from build123d import *

# Parameters (mm, degrees)
SKETCH1_W                     = 320
SKETCH1_H                     = 50
BOSS_EXTRUDE1_DEPTH           = 4
M5_CLEARANCE_HOLE1_AT_2_COUNT = 2
M5_CLEARANCE_HOLE1_AT_2_PITCH = 300
LPATTERN1_COUNT               = 2
LPATTERN1_PITCH               = 25
SKETCH5_W                     = 80
SKETCH5_H                     = 15
CUT_EXTRUDE1_DEPTH            = 324.907394173
CUT_EXTRUDE3_DEPTH            = 324.907394173
M2_5_CLEARANCE_HOLE1_D        = 2.9
M2_5_CLEARANCE_HOLE1_DEPTH    = 14
M2_5_CLEARANCE_HOLE1_TIP      = 0.871247898
DRAFT1_ANGLE                  = -20


with BuildPart() as part:
    # Sketch1 → Boss-Extrude1 (new body)
    with BuildSketch(Plane.XY):
        with Locations((160, 25)):
            Rectangle(SKETCH1_W, SKETCH1_H)
    extrude(amount=BOSS_EXTRUDE1_DEPTH)

    # Sketch4 → M5 Clearance Hole1 (revolve, cut)
    with BuildSketch(Plane(origin=(310, 37.5, 4), x_dir=(0, -1, 0), z_dir=(1, 0, 0))):
        Polygon((0, 0), (0, 15.652366702), (2.75, 14), (2.75, 0), align=None)
    m5_clearance_hole1 = revolve(axis=Axis((310, 37.5, 10.35), (0, 0, -1)), mode=Mode.SUBTRACT)

    # M5 Clearance Hole1 at 2: M5 Clearance Hole1 ×2
    with Locations(*[(-i * M5_CLEARANCE_HOLE1_AT_2_PITCH, 0, 0) for i in range(1, M5_CLEARANCE_HOLE1_AT_2_COUNT)]):
        add(m5_clearance_hole1, mode=Mode.SUBTRACT)

    # LPattern1: M5 Clearance Hole1 ×2
    with Locations(*[(0, -i * LPATTERN1_PITCH, 0) for i in range(1, LPATTERN1_COUNT)]):
        add(m5_clearance_hole1, mode=Mode.SUBTRACT)

    # LPattern1 copy 1 sketch → LPattern1 copy 1 (revolve, cut)
    with BuildSketch(Plane(origin=(10, 12.5, 4), x_dir=(0, -1, 0), z_dir=(1, 0, 0))):
        Polygon((0, 0), (0, 15.652366702), (2.75, 14), (2.75, 0), align=None)
    revolve(axis=Axis((10, 12.5, 10.35), (0, 0, -1)), mode=Mode.SUBTRACT)

    # Sketch5 → Cut-Extrude1 (cut, through all)
    with BuildSketch(Plane.XY.offset(4)):
        with Locations((105, 25)):
            Rectangle(SKETCH5_W, SKETCH5_H)
    extrude(amount=-CUT_EXTRUDE1_DEPTH, mode=Mode.SUBTRACT)

    # Sketch6 → Cut-Extrude3 (cut, through all)
    with BuildSketch(Plane.XY.offset(4)):
        with BuildLine():
            Line((27, 24.6), (27, 33))
            ThreePointArc((27, 33), (31, 37), (35, 33))
            Line((35, 33), (35, 24.6))
            ThreePointArc((35, 24.6), (31, 20.6), (27, 24.6))
        make_face()
    extrude(amount=-CUT_EXTRUDE3_DEPTH, mode=Mode.SUBTRACT)

    # M2.5 Clearance Hole1
    with Locations(Plane.XY.offset(4)):
        with Locations((140, 5.6), (26, 5.6), (36, 5.6), (70, 5.6)):
            Hole(M2_5_CLEARANCE_HOLE1_D / 2, depth=M2_5_CLEARANCE_HOLE1_DEPTH)
            with Locations((0, 0, -(M2_5_CLEARANCE_HOLE1_DEPTH + M2_5_CLEARANCE_HOLE1_TIP / 2))):  # 118° drill point
                Cone(0, M2_5_CLEARANCE_HOLE1_D / 2, M2_5_CLEARANCE_HOLE1_TIP, mode=Mode.SUBTRACT)

    # Draft1
    draft1_faces = [part.faces().sort_by_distance(p)[0] for p in [
        (145, 25, 2),
        (105, 32.5, 2),
        (65, 25, 2),
        (105, 17.5, 2),
        (35, 28.8, 2),
        (31, 37, 2),
        (27, 28.8, 2),
        (31, 20.6, 2),
    ]]
    draft(draft1_faces, Plane(origin=(0, 0, 0), x_dir=(-1, 0, 0), z_dir=(0, 0, -1)), DRAFT1_ANGLE)


solid = part.part
For this review, take the finished solid that the model builds, in its own axes (mm). A direction names the side the tool comes from. Give positions to 0.01 mm unless a question says otherwise; leave off trailing zeros. Order: outer loops, then holes, each group sorted by start corner. A loop starts at its lowest first (then second) coordinate and runs counter-clockwise, first axis right, second up. Notation, with made-up numbers: (-37.5, 36.5) - (-18.5, 36.5) arc R12 ccw to (-18.5, 43.5) - close; hole circle Ø11 at (53.5, -31). An arc over 180 degrees is marked (long way). Answer as a JSON object with one key per item and string values. Group by question number.
Item 1: Take a section at D-D on x = 88. Give the boundary of the cut face in (y, z), and give its area (3 significant figures).
Item 2: Draft analysis for pull direction X (two halves, no side actions). For faces 1 (the conical face through (31.101, 20.025, 1.584)), 2 (the flat face through (158, 25, 4)), state which applies: pulls with the +X half, pulls with the -X half, needs draft (parallel to the pull), parting line crosses it, or undercut.
Item 3: Take a section at C-C on z = 3.3. Give the number of separate pieces and of enclosed holes in the cut face, and give its area (3 significant figures).
Item 4: Machinability: for faces 3 (the flat face through (158, 25, 0)), 4 (the conical face through (30.899, 37.575, 1.584)), which of the approach directions +Z, -Z, +X, -X, +Y, -Y give a long, thin tool a straight path to every point of the face, cutting with its end or side? Answer none if there is none.
Item 5: Take a section at A-A on x = 31. Give the boundary of the cut face in (y, z), and give its area (3 significant figures).
Item 6: Wall thickness on line 1 along Y through (x, z) = (10, 1.35); line 2 along Y through (x, z) = (26, 2.15); line 3 along X through (y, z) = (35, 3.7): over which ranges is each line inside the solid? List them lowest first.
Item 7: Take a section at B-B on y = 12.5. Give the boundary of the cut face in (x, z), and give its area (3 significant figures).
Item 8: Clearance check with a flat-ended pin moving along its axis: pin 1 Ø1.5 at (x, y) = (90.5, 31) entering from -Z. State where the tip first meets the part, or that it passes through.
Reported:
{
 "1": {"outline": "(0, 0) - (17.5, 0) - (16.04, 4) - (0, 4) - close; (32.5, 0) - (50, 0) - (50, 4) - (33.96, 4) - close", "area": "134 mm^2"},
 "2": {"face 1": "undercut", "face 2": "needs draft"},
 "3": {"separate pieces": "1", "enclosed holes": "10", "area": "14,300 mm^2"},
 "4": {"face 3": "-Z, +X, -X, +Y, -Y", "face 4": "+Z"},
 "5": {"outline": "(0, 0) - (20.6, 0) - (19.14, 4) - (0, 4) - close; (37, 0) - (50, 0) - (50, 4) - (38.46, 4) - close", "area": "129 mm^2"},
 "6": {"line 1": "0 to 9.75, 15.25 to 34.75, 40.25 to 50", "line 2": "0 to 4.15, 7.05 to 50", "line 3": "0 to 8.85, 11.15 to 26.04, 35.96 to 308.85, 311.15 to 320"},
 "7": {"outline": "(0, 0) - (7.25, 0) - (7.25, 4) - (0, 4) - close; (12.75, 0) - (307.25, 0) - (307.25, 4) - (12.75, 4) - close; (312.75, 0) - (320, 0) - (320, 4) - (312.75, 4) - close", "area": "1,240 mm^2"},
 "8": {"pin 1": "through"}
}
